Can you work these out from the model? Positions are in its coordinate system, mm. Face numbers are marked on the shaded views. Round coordinates to 2 decimals unless told otherwise and drop trailing zeros. Order: outer loops, then holes, each group sorted by start corner. A loop starts at its lowest first (then second) coordinate and runs counter-clockwise, first axis right, second up. Notation, with made-up numbers: M -18.5,2 L -10.5,2 A16 cw -10.5,33 Z; hole C -29,-20.75 d2. An arc over 180 degrees is marked long. Answer as a JSON object with one key per item and string values. Group by question number.
Autodesk Inventor part; units mm, degrees
ref_plane "YZ Plane" through (0, 0, 0) normal (1, 0, 0) x (0, 1, 0)
ref_plane "XZ Plane" through (0, 0, 0) normal (0, 1, 0) x (-1, 0, 0)
ref_plane "XY Plane" through (0, 0, 0) normal (0, 0, 1) x (1, 0, 0)
sketch "Sketch1" plane through (0, 0, 0) normal (0, 1, 0) x (-1, 0, 0)
  circle A0 centre (0, 0) radius 54
  circle A1 centre (0, 0) radius 57
  dimension "d0" = 3
  dimension "d1" = 114
extrude "Extrusion1" add sketch "Sketch1" along normal blind 200
sketch "Sketch2" plane through (0, 200, 0) normal (0, 1, 0) x (1, 0, 0)
  circle A0 centre (0, 0) radius 57
  line L0 (55.9285, -11) -> (-55.9285, -11)
  line L1 (-55.9285, -11) -> (-55.9285, 11)
  line L2 (-55.9285, 11) -> (55.9285, 11)
  line L3 (55.9285, 11) -> (55.9285, -11)
  line L4 (55.9285, -11) -> (-55.9285, 11) construction
  line L5 (-55.9285, -11) -> (55.9285, 11) construction
  dimension "d4" = 22
extrude "Extrusion2" cut sketch "Sketch2" against normal blind 20 contours A0 L3 | L1 A0
sketch "Sketch3" plane through (-55.9285, 200, -11) normal (-1, 0, 0) x (0, 0, 1)
  line L0 (0, -20) -> (22, -20)
  line L1 (16, -20) -> (6, -20)
  line L2 (6, -20) -> (6, 20)
  line L3 (6, 20) -> (16, 20)
  line L4 (16, 20) -> (16, -20)
  line L5 (0, -20) -> (0, 0)
  point P0 (11, -200)
  point P1 (6, 0)
  point P2 (6, -20)
  dimension "d7" = 40
  dimension "d8" = 10
  dimension "d9" = 6
extrude "Extrusion3" add sketch "Sketch3" along normal blind 10
mirror "Mirror1" about plane through (0, 0, 0) normal (1, 0, 0) of "Extrusion3"
sketch "Sketch4" plane through (0, 0, 0) normal (0, -1, 0) x (1, 0, 0)
  line L0 (-2.5, -60) -> (2.5, -60)
  line L1 (2.5, -60) -> (2.5, 60)
  line L2 (2.5, 60) -> (-2.5, 60)
  line L3 (-2.5, 60) -> (-2.5, -60)
  line L4 (-2.5, -60) -> (2.5, 60) construction
  line L5 (2.5, -60) -> (-2.5, 60) construction
  line L6 (60, -2.5) -> (-60, -2.5)
  line L7 (-60, -2.5) -> (-60, 2.5)
  line L8 (-60, 2.5) -> (60, 2.5)
  line L9 (60, 2.5) -> (60, -2.5)
  line L10 (60, -2.5) -> (-60, 2.5) construction
  line L11 (-60, -2.5) -> (60, 2.5) construction
  point P0 (0, 0)
  point P1 (-2.5, -2.5)
  point P2 (2.5, -2.5)
  point P3 (2.5, 2.5)
  point P4 (-2.5, 2.5)
  dimension "d12" = 5
  dimension "d13" = 5
  dimension "d14" = 120
  dimension "d15" = 120
extrude "Extrusion4" cut sketch "Sketch4" against normal blind 10
equation "\"d13\" = d12"
equation "\"d15\" = d14"
properties part number "Cooking Pipe"
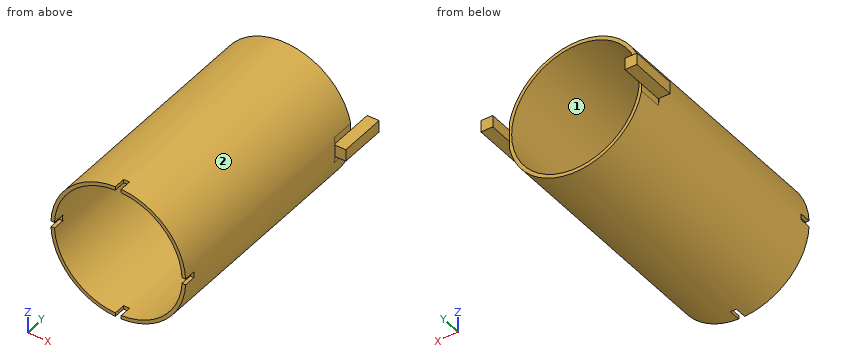
Item 1: Suppose I cut it at B-B, the plane x = 0. Write out the boundary of the cut face in (y, z), and give its area (3 significant figures).
Item 2: Suppose I cut it at A-A, the plane z = 0. Write out the boundary of the cut face in (x, y).
Item 3: If we mould it in two halves opening along Z, with no side actions, what happens to the marked faces 1 and 2? For each: +Z half, -Z half, draft (parallel to the pull), parting line (faces both ways), or undercut.
Item 4: Suppose I cut it at C-C, the plane y = 149. Write out the boundary of the cut face in (x, z).
Item 5: I'm going to push flat-ended pins straight in: pin 1 Ø3.5 at (x, z) = (55.5, 1) entering from -Y; pin 2 Ø0.7 at (x, z) = (56, -9) entering from +Y; pin 3 Ø10 at (x, z) = (-47, 13.5) entering from -Y; pin 4 Ø12 at (x, y) = (-19, 80.5) entering from -Z. Where does each tip first touch, or does it pass through?
Item 6: Suppose I cut it at D-D, the plane x = -41. Write out the boundary of the cut face in (y, z).
Item 7: I need wall thicknesses on line 1 (Z direction, x = 0, y = 152); line 2 (X direction, y = 190, z = 23). Which ranges of each line are inside material? Lowest first, please.
Computed:
{
 "1": {"outline": "M 10,-57 L 200,-57 L 200,-54 L 10,-54 Z; M 10,54 L 200,54 L 200,57 L 10,57 Z", "area": "1,140 mm^2"},
 "2": {"outline": "M -65.93,180 L -57,180 L -57,10 L -54,10 L -54,200 L -55.93,200 L -55.93,220 L -65.93,220 Z; M 54,10 L 57,10 L 57,180 L 65.93,180 L 65.93,220 L 55.93,220 L 55.93,200 L 54,200 Z"},
 "3": {"face 1": "undercut", "face 2": "parting line"},
 "4": {"outline": "C 0,0 d114; hole C 0,0 d108"},
 "5": {"pin 1": "stops at y = 0", "pin 2": "stops at y = 200", "pin 3": "passes through", "pin 4": "stops at z = -55.5"},
 "6": {"outline": "M 0,-39.6 L 200,-39.6 L 200,-35.14 L 0,-35.14 Z; M 0,35.14 L 200,35.14 L 200,39.6 L 0,39.6 Z"},
 "7": {"line 1": "z = -57 to -54, 54 to 57", "line 2": "x = -52.15 to -48.86, 48.86 to 52.15"}
}
